Work out the finished part from the listing and answer in its coordinate system (mm). A direction names the side the tool comes from. Give positions to 0.01 mm unless a question says otherwise; leave off trailing zeros. Write each loop counter-clockwise with the first axis right and the second up, starting at its lowest first coordinate (ties: lowest second). Pieces come first, ordered by that corner, then holes. Notation, with made-up numbers: (36, 83.5) - (55, 83.5) arc R17 cw to (55, 87.5) - close; hole circle Ø6 at (-40, -17.75). An arc over 180 degrees is marked (long way). Write item = value, one per line.
from build123d import *

# Parameters (mm, degrees)
BOSS_EXTRUDE1_DEPTH = 279.4
SKETCH2_R           = 3.1877
CUT_EXTRUDE1_DEPTH  = 280.656768379


with BuildPart() as part:
    # Sketch1 → Boss-Extrude1 (new body)
    with BuildSketch(Plane.XY):
        Polygon((-10.16, 0), (-10.16, 6.35), (10.16, 6.35), (10.16, 0), (9.7536, 0), (9.7536, 5.9436), (-9.7536, 5.9436), (-9.7536, 0), align=None)
    extrude(amount=-BOSS_EXTRUDE1_DEPTH)

    # Sketch2 → Cut-Extrude1 (cut, through all)
    with BuildSketch(Plane(origin=(0, 6.35, 0), x_dir=(1, 0, 0), z_dir=(0, 1, 0))):
        with Locations(Location((0, 266.7, 0), (0, 0, 270))):
            Circle(SKETCH2_R)
        with Locations(Location((0, 12.7, 0), (0, 0, 270))):
            Circle(SKETCH2_R)
    extrude(amount=-CUT_EXTRUDE1_DEPTH, mode=Mode.SUBTRACT)


solid = part.part
1. Given pin 1 (1 mm diameter, centred on x = -5.5, y = 4.5, fed in from +Z); pin 2 (2 mm diameter, centred on x = -0.5, z = -124.5, fed in from -Y), each flat-ended and moving along its own axis, determine where each tip first touches the part or whether it passes through.
Solution:
pin_1 = through
pin_2 = 5.94
2. For a pull along X with two mould halves and no side action, classify faces 3 (the flat face through (-10.16, 3, -138)), 4 (the flat face through (10.16, 3, -138)), 5 (the flat face through (0, 6.35, -138)), 6 (the flat face through (0, 5.944, -138)) as pulls with the +X half, pulls with the -X half, needs draft (parallel to the pull), parting line crosses it, or undercut.
Solution:
face_3 = pulls with the -X half
face_4 = pulls with the +X half
face_5 = needs draft
face_6 = undercut
3. A tool of negligible diameter and unlimited length cuts with its end or side. For faces 1 (the cylindrical face through (-1.221, 6.15, -263.755)), 2 (the flat face through (9.754, 3, -138)), from which of +Z, -Z, +X, -X, +Y, -Y can it reach the whole face along a straight path? Write none if from no direction.
Solution:
face_1 = +Y, -Y
face_2 = +Z, -Z, -Y
4. Find section A-A, the plane y = 1. Give the vertices of the cut face in (x, z).
Solution:
outline = (-10.16, -279.4) - (-9.75, -279.4) - (-9.75, 0) - (-10.16, 0) - close; (9.75, -279.4) - (10.16, -279.4) - (10.16, 0) - (9.75, 0) - close
5. Find section C-C, the plane x = 0. Give the vertices of the cut face in (y, z).
Solution:
outline = (5.94, -279.4) - (6.35, -279.4) - (6.35, -269.89) - (5.94, -269.89) - close; (5.94, -263.51) - (6.35, -263.51) - (6.35, -15.89) - (5.94, -15.89) - close; (5.94, -9.51) - (6.35, -9.51) - (6.35, 0) - (5.94, 0) - close
6. Straight lines are drawn through the part: line 1 (X direction, y = 6.15, z = -266.7); line 2 (X direction, y = 5.5, z = -190); line 3 (Y direction, x = -4.25, z = -209). For each, find the intervals that lie inside material, in ascending order.
Solution:
line_1 = -10.16 to -3.19, 3.19 to 10.16
line_2 = -10.16 to -9.75, 9.75 to 10.16
line_3 = 5.94 to 6.35
7. Find section D-D, the plane z = -104.5. Give the vertices of the cut face in (x, y), then the cut area to 3 significant figures.
Solution:
outline = (-10.16, 0) - (-9.75, 0) - (-9.75, 5.94) - (9.75, 5.94) - (9.75, 0) - (10.16, 0) - (10.16, 6.35) - (-10.16, 6.35) - close
area = 13.1 mm^2
8. Find section B-B, the plane z = -12.7. Give the vertices of the cut face in (x, y), then the cut area to 3 significant figures.
Solution:
outline = (-10.16, 0) - (-9.75, 0) - (-9.75, 5.94) - (-3.19, 5.94) - (-3.19, 6.35) - (-10.16, 6.35) - close; (3.19, 5.94) - (9.75, 5.94) - (9.75, 0) - (10.16, 0) - (10.16, 6.35) - (3.19, 6.35) - close
area = 10.5 mm^2
